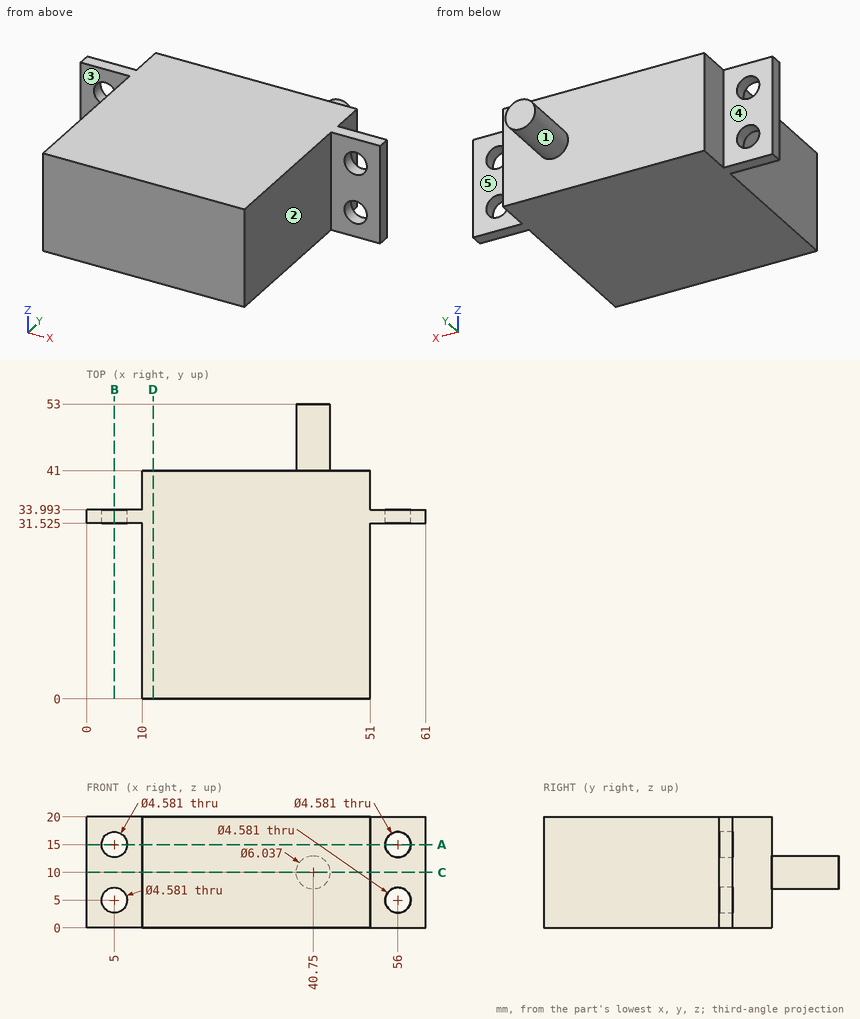
Could you check a few things on this drawing? It's one solid part, dimensions in mm from its lowest x, y, z. A direction names the side the tool comes from. Coordinates: 2 decimals unless noted, no trailing zeros. Order: outer loops, then holes, each group sorted by start corner. A loop starts at its lowest first (then second) coordinate and runs counter-clockwise, first axis right, second up. Notation, with made-up numbers: (-6.75, -11) - (-2.75, -11) arc R31 ccw to (-2.75, 28) - close; hole circle Ø4 at (27.25, 37.5). An arc over 180 degrees is marked (long way). One line per question, with ' | ' between items.
(1) For the marked faces 1, 2, 3, 4 and 5, which set-ups out of +Z, -Z, +X, -X, +Y, -Y let a thin tool reach every point of the face, with its end or its side?
Report:
face 1: +Y | face 2: +Z, -Z, +X, -Y | face 3: +Z, -Z, -X, -Y | face 4: +Z, -Z, -X, +Y | face 5: +Z, -Z, +X, +Y
(2) Suppose I cut it at D-D on x = 12. List the corners of the cut face in (y, z) for me.
Report:
outline: (0, 0) - (41, 0) - (41, 20) - (0, 20) - close
(3) Suppose I cut it at C-C on z = 10. List the corners of the cut face in (x, y) for me (1 decimal).
Report:
outline: (0, 31.5) - (10, 31.5) - (10, 0) - (51, 0) - (51, 31.5) - (61, 31.5) - (61, 34) - (51, 34) - (51, 41) - (43.8, 41) - (43.8, 53) - (37.7, 53) - (37.7, 41) - (10, 41) - (10, 34) - (0, 34) - close
(4) If I drill on L1, parallel to X at y = 32.2, z = 15; L2, parallel to Z at x = 56, y = 32.85; L3, parallel to Y at x = 29, z = 5.5, over which ranges is the centre line in solid material (lowest first)?
Report:
L1: x = 0 to 2.71, 7.29 to 53.71, 58.29 to 61 | L2: z = 0 to 2.71, 7.29 to 12.71, 17.29 to 20 | L3: y = 0 to 41
(5) Will these pins go through, and if not, where does the flat tip stop? pin 1 (3.5 mm diameter, centred on y = 37, z = 12, fed in from +X); pin 2 (6 mm diameter, centred on x = 56, z = 15, fed in from +Y); pin 3 (10 mm diameter, centred on x = 15.5, z = 6.5, fed in from +Y).
Report:
pin 1: stops at x = 51 | pin 2: stops at y = 33.99 | pin 3: stops at y = 41
(6) Suppose I cut it at A-A on z = 15. List the corners of the cut face in (x, y) for me (1 decimal), and give its area (3 significant figures).
Report:
outline: (0, 31.5) - (2.7, 31.5) - (2.7, 34) - (0, 34) - close; (7.3, 31.5) - (10, 31.5) - (10, 0) - (51, 0) - (51, 31.5) - (53.7, 31.5) - (53.7, 34) - (51, 34) - (51, 41) - (10, 41) - (10, 34) - (7.3, 34) - close; (58.3, 31.5) - (61, 31.5) - (61, 34) - (58.3, 34) - close | area: 1,710 mm2
(7) Suppose I cut it at B-B on x = 5. List the corners of the cut face in (y, z) for me (1 decimal).
Report:
outline: (31.5, 0) - (34, 0) - (34, 2.7) - (31.5, 2.7) - close; (31.5, 7.3) - (34, 7.3) - (34, 12.7) - (31.5, 12.7) - close; (31.5, 17.3) - (34, 17.3) - (34, 20) - (31.5, 20) - close
